```python
from build123d import *

# Parameters (mm, degrees)
SZKIC1_W                     = 24
SZKIC1_H                     = 52
DODANIE_WYCI_GNI_CIE1_DEPTH  = 25
SZKIC2_W                     = 26
SZKIC2_H                     = 54
SZKIC2_W_2                   = 21
SZKIC2_H_2                   = 49
DODANIE_WYCI_GNI_CIE2_DEPTH  = 12
SZKIC3_W                     = 38
SZKIC3_H                     = 54
SZKIC3_W_2                   = 21
SZKIC3_H_2                   = 49
DODANIE_WYCI_GNI_CIE3_DEPTH  = 2
SZKIC4_W                     = 38
SZKIC4_H                     = 54
DODANIE_WYCI_GNI_CIE4_DEPTH  = 3
ZAOKR_GLENIE1_R              = 3.5
SZKIC5_R                     = 1.5
DODANIE_WYCI_GNI_CIE9_DEPTH  = 3
WYTNIJ_WYCI_GNI_CIE2_REACH   = 63.425
SZKIC7_W                     = 20
SZKIC7_H                     = 11
SZKIC8_W                     = 34
SZKIC8_H                     = 96
SZKIC8_W_2                   = 30
SZKIC8_H_2                   = 92
DODANIE_WYCI_GNI_CIE5_DEPTH  = 18.5
SZKIC9_W                     = 34
SZKIC9_H                     = 96
DODANIE_WYCI_GNI_CIE6_DEPTH  = 3
SZKIC10_R                    = 1.9
WYTNIJ_WYCI_GNI_CIE3_DEPTH   = 70.873099259
ZAOKR_GLENIE2_R              = 4
SZKIC11_W                    = 34
SZKIC11_H                    = 96
SZKIC11_R                    = 4
DODANIE_WYCI_GNI_CIE7_DEPTH  = 3.5
SZKIC20_R                    = 4
DODANIE_WYCI_GNI_CIE10_DEPTH = 10
SZKIC21_R                    = 4
DODANIE_WYCI_GNI_CIE11_DEPTH = 5
SZKIC13_R                    = 1.5
WYTNIJ_WYCI_GNI_CIE4_DEPTH   = 6
WYTNIJ_WYCI_GNI_CIE5_DEPTH   = 72.028163428
SFAZOWANIE1_SIZE             = 0.5
SFAZOWANIE2_SIZE             = 2.1
ZAOKR_GLENIE3_R              = 6
ZAOKR_GLENIE4_R              = 4
SZKIC18_R                    = 3.5
WYTNIJ_WYCI_GNI_CIE8_DEPTH   = 10
SFAZOWANIE3_SIZE             = 1.5
SZKIC19_R                    = 2
WYTNIJ_WYCI_GNI_CIE9_DEPTH   = 73.938330286
WYTNIJ_WYCI_GNI_CIE10_REACH  = 92.161
SZKIC22_W                    = 15
SZKIC22_H                    = 9
ZAOKR_GLENIE5_R              = 3


with BuildPart() as part:
    # Szkic1 → Dodanie-wyciągnięcie1 (new body)
    with BuildSketch(Plane(origin=(0, 0, 0), x_dir=(1, 0, 0), z_dir=(0, 1, 0))):
        Rectangle(SZKIC1_W, SZKIC1_H)
        with BuildLine():
            Line((10, 14.5), (10, -14.5))
            ThreePointArc((10, -14.5), (0, -24.5), (-10, -14.5))
            Line((-10, -14.5), (-10, 14.5))
            ThreePointArc((-10, 14.5), (0, 24.5), (10, 14.5))
        make_face(mode=Mode.SUBTRACT)
    extrude(amount=DODANIE_WYCI_GNI_CIE1_DEPTH)

    # Szkic2 → Dodanie-wyciągnięcie2 (add)
    with BuildSketch(Plane(origin=(0, 25, 0), x_dir=(1, 0, 0), z_dir=(0, 1, 0))):
        Rectangle(SZKIC2_W, SZKIC2_H)
        Rectangle(SZKIC2_W_2, SZKIC2_H_2, mode=Mode.SUBTRACT)
    extrude(amount=DODANIE_WYCI_GNI_CIE2_DEPTH)

    # Szkic3 → Dodanie-wyciągnięcie3 (add)
    with BuildSketch(Plane(origin=(0, 37, 0), x_dir=(1, 0, 0), z_dir=(0, 1, 0))):
        Rectangle(SZKIC3_W, SZKIC3_H)
        Rectangle(SZKIC3_W_2, SZKIC3_H_2, mode=Mode.SUBTRACT)
    extrude(amount=-DODANIE_WYCI_GNI_CIE3_DEPTH)

    # Szkic4 → Dodanie-wyciągnięcie4 (add)
    with BuildSketch(Plane(origin=(0, 37, 0), x_dir=(1, 0, 0), z_dir=(0, 1, 0))):
        Rectangle(SZKIC4_W, SZKIC4_H)
        Polygon((-10, 24.5), (10, 24.5), (10.5, 24.5), (10.5, 18.35), (18, 18.35), (18, 10.35), (10.5, 10.35), (10.5, -10.35), (18, -10.35), (18, -18.35), (10.5, -18.35), (10.5, -24.5), (10, -24.5), (-10, -24.5), (-10.5, -24.5), (-10.5, -18.35), (-18, -18.35), (-18, -10.35), (-10.5, -10.35), (-10.5, 10.35), (-18, 10.35), (-18, 18.35), (-10.5, 18.35), (-10.5, 24.5), align=None, mode=Mode.SUBTRACT)
    extrude(amount=DODANIE_WYCI_GNI_CIE4_DEPTH)

    # Zaokrąglenie1
    zaokr_glenie1_edges = [part.edges().sort_by_distance(p)[0] for p in [
        (10.5, 38.5, -18.35),
        (18, 38.5, -18.35),
        (18, 38.5, -10.35),
        (10.5, 38.5, -10.35),
        (10.5, 38.5, 10.35),
        (18, 38.5, 10.35),
        (18, 38.5, 18.35),
        (10.5, 38.5, 18.35),
        (-10.5, 38.5, 18.35),
        (-18, 38.5, 18.35),
        (-18, 38.5, 10.35),
        (-10.5, 38.5, 10.35),
        (-10.5, 38.5, -10.35),
        (-18, 38.5, -10.35),
        (-18, 38.5, -18.35),
        (-10.5, 38.5, -18.35),
    ]]
    fillet(zaokr_glenie1_edges, radius=ZAOKR_GLENIE1_R)

    # Szkic5 → Dodanie-wyciągnięcie9 (add)
    with BuildSketch(Plane(origin=(0, 37, 0), x_dir=(1, 0, 0), z_dir=(0, 1, 0))):
        with Locations(Location((13.85, -14.35, 0), (0, 0, 270))):
            Circle(SZKIC5_R)
        with Locations(Location((13.85, 14.35, 0), (0, 0, 270))):
            Circle(SZKIC5_R)
        with Locations(Location((-13.85, -14.35, 0), (0, 0, 90))):
            Circle(SZKIC5_R)
        with Locations(Location((-13.85, 14.35, 0), (0, 0, 90))):
            Circle(SZKIC5_R)
    extrude(amount=DODANIE_WYCI_GNI_CIE9_DEPTH)

    # Szkic7 → Wytnij-wyciągnięcie2 (cut, up to next)
    with BuildSketch(Plane.ZY.offset(19), mode=Mode.PRIVATE) as wytnij_wyci_gni_cie2_sk1:
        with Locations((0, 32)):
            Rectangle(SZKIC7_W, SZKIC7_H)
    wytnij_wyci_gni_cie2_tool1 = extrude(wytnij_wyci_gni_cie2_sk1.sketch, amount=-WYTNIJ_WYCI_GNI_CIE2_REACH, mode=Mode.PRIVATE) & part.part
    add(wytnij_wyci_gni_cie2_tool1.solids().sort_by_distance((-19, 32, 0))[0], mode=Mode.SUBTRACT)

    # Szkic8 → Dodanie-wyciągnięcie5 (add)
    with BuildSketch(Plane(origin=(0, 0, 0), x_dir=(1, 0, 0), z_dir=(0, 1, 0))):
        with Locations((29, 0)):
            Rectangle(SZKIC8_W, SZKIC8_H)
        with Locations((29, 0)):
            Rectangle(SZKIC8_W_2, SZKIC8_H_2, mode=Mode.SUBTRACT)
    extrude(amount=DODANIE_WYCI_GNI_CIE5_DEPTH)

    # Szkic9 → Dodanie-wyciągnięcie6 (add)
    with BuildSketch(Plane(origin=(0, 18.5, 0), x_dir=(1, 0, 0), z_dir=(0, 1, 0))):
        with Locations((29, 0)):
            Rectangle(SZKIC9_W, SZKIC9_H)
    extrude(amount=DODANIE_WYCI_GNI_CIE6_DEPTH)

    # Szkic10 → Wytnij-wyciągnięcie3 (cut, through all)
    with BuildSketch(Plane(origin=(0, 21.5, 0), x_dir=(1, 0, 0), z_dir=(0, 1, 0))):
        with Locations(Location((24.5, 37.5, 0), (0, 0, 270))):
            Circle(SZKIC10_R)
        with Locations(Location((24.5, -37.5, 0), (0, 0, 270))):
            Circle(SZKIC10_R)
    extrude(amount=-WYTNIJ_WYCI_GNI_CIE3_DEPTH, mode=Mode.SUBTRACT)

    # Zaokrąglenie2
    zaokr_glenie2_edges = [part.edges().sort_by_distance(p)[0] for p in [
        (44, 9.25, -46),
        (14, 9.25, -46),
        (14, 9.25, 46),
        (44, 9.25, 46),
    ]]
    fillet(zaokr_glenie2_edges, radius=ZAOKR_GLENIE2_R)

    # Szkic11 → Dodanie-wyciągnięcie7 (add)
    with BuildSketch(Plane(origin=(0, 21.5, 0), x_dir=(1, 0, 0), z_dir=(0, 1, 0))):
        with Locations((29, 0)):
            Rectangle(SZKIC11_W, SZKIC11_H)
        with Locations(Location((24.5, 37.5, 0), (0, 0, 90))):
            Circle(SZKIC11_R, mode=Mode.SUBTRACT)
        with Locations(Location((24.5, -37.5, 0), (0, 0, 90))):
            Circle(SZKIC11_R, mode=Mode.SUBTRACT)
    extrude(amount=DODANIE_WYCI_GNI_CIE7_DEPTH)

    # Szkic20 → Dodanie-wyciągnięcie10 (add)
    with BuildSketch(Plane(origin=(0, 25, 0), x_dir=(1, 0, 0), z_dir=(0, 1, 0))):
        Polygon((12, 27), (13, 27), (13, -27), (12, -27), (12, -48), (46, -48), (46, 48), (12, 48), align=None)
        with Locations(Location((24.5, 37.5, 0), (0, 0, 90))):
            Circle(SZKIC20_R, mode=Mode.SUBTRACT)
        with Locations(Location((24.5, -37.5, 0), (0, 0, 90))):
            Circle(SZKIC20_R, mode=Mode.SUBTRACT)
    extrude(amount=DODANIE_WYCI_GNI_CIE10_DEPTH)

    # Szkic21 → Dodanie-wyciągnięcie11 (add)
    with BuildSketch(Plane(origin=(0, 35, 0), x_dir=(1, 0, 0), z_dir=(0, 1, 0))):
        Polygon((12, 27), (19, 27), (19, -27), (12, -27), (12, -48), (46, -48), (46, 48), (12, 48), align=None)
        with Locations(Location((24.5, 37.5, 0), (0, 0, 90))):
            Circle(SZKIC21_R, mode=Mode.SUBTRACT)
        with Locations(Location((24.5, -37.5, 0), (0, 0, 90))):
            Circle(SZKIC21_R, mode=Mode.SUBTRACT)
    extrude(amount=DODANIE_WYCI_GNI_CIE11_DEPTH)

    # Szkic13 → Wytnij-wyciągnięcie4 (cut)
    with BuildSketch(Plane(origin=(0, 40, 0), x_dir=(1, 0, 0), z_dir=(0, 1, 0))):
        with Locations(Location((41.5, 33, 0), (0, 0, 270))):
            Circle(SZKIC13_R)
        with Locations(Location((41.5, -33, 0), (0, 0, 270))):
            Circle(SZKIC13_R)
        with Locations(Location((16.5, -33, 0), (0, 0, 90))):
            Circle(SZKIC13_R)
        with Locations(Location((16.5, 33, 0), (0, 0, 90))):
            Circle(SZKIC13_R)
        with Locations(Location((29, 0, 0), (0, 0, 270))):
            Circle(SZKIC13_R)
    extrude(amount=-WYTNIJ_WYCI_GNI_CIE4_DEPTH, mode=Mode.SUBTRACT)

    # Szkic14 → Wytnij-wyciągnięcie5 (cut, through all)
    with BuildSketch(Plane(origin=(0, 25, 0), x_dir=(1, 0, 0), z_dir=(0, 1, 0))):
        Polygon((10, 0), (10, 18.642135624), (4.142135624, 24.5), (-4.142135624, 24.5), (-10, 18.642135624), (-10, 0), (-10, -18.642135624), (-4.142135624, -24.5), (4.142135624, -24.5), (10, -18.642135624), align=None)
    extrude(amount=-WYTNIJ_WYCI_GNI_CIE5_DEPTH, mode=Mode.SUBTRACT)

    # Sfazowanie1
    sfazowanie1_edges = [part.edges().sort_by_distance(p)[0] for p in [
        (10.5, 25, 0),
        (-10.5, 25, 0),
    ]]
    chamfer(sfazowanie1_edges, length=SFAZOWANIE1_SIZE - 0.0001)  # a hair under: the kernel refuses the full size

    # Sfazowanie2
    sfazowanie2_edges = [part.edges().sort_by_distance(p)[0] for p in [
        (24.5, 21.5, -33.5),
        (24.5, 21.5, 41.5),
    ]]
    chamfer(sfazowanie2_edges, length=SFAZOWANIE2_SIZE - 0.0001)  # a hair under: the kernel refuses the full size

    # Zaokrąglenie3
    zaokr_glenie3_edges = [part.edges().sort_by_distance(p)[0] for p in [
        (12, 12.5, 26),
        (12, 12.5, -26),
        (-19, 37.5, 27),
        (-19, 37.5, -27),
        (-12, 12.5, -26),
        (-12, 12.5, 26),
        (12, 20, -48),
        (46, 20, -48),
        (46, 20, 48),
        (12, 20, 48),
        (-13, 30, -27),
        (-13, 30, 27),
    ]]
    fillet(zaokr_glenie3_edges, radius=ZAOKR_GLENIE3_R)

    # Zaokrąglenie4
    zaokr_glenie4_edges = [part.edges().sort_by_distance(p)[0] for p in [
        (-15.737192685, 37.5, 10),
        (-15.737192685, 37.5, -10),
    ]]
    fillet(zaokr_glenie4_edges, radius=ZAOKR_GLENIE4_R)

    # Szkic18 → Wytnij-wyciągnięcie8 (cut)
    with BuildSketch(Plane(origin=(0, 40, 0), x_dir=(1, 0, 0), z_dir=(0, 1, 0))):
        with Locations((47, 40)):
            Circle(SZKIC18_R)
        with Locations((47, -40)):
            Circle(SZKIC18_R)
    extrude(amount=-WYTNIJ_WYCI_GNI_CIE8_DEPTH, mode=Mode.SUBTRACT)

    # Sfazowanie3
    sfazowanie3_edges = [part.edges().sort_by_distance(p)[0] for p in [
        (43.500820064, 30, -39.924238715),
        (43.500820064, 30, 39.924238715),
    ]]
    chamfer(sfazowanie3_edges, length=SFAZOWANIE3_SIZE)

    # Szkic19 → Wytnij-wyciągnięcie9 (cut, through all)
    with BuildSketch(Plane(origin=(0, 30, 0), x_dir=(1, 0, 0), z_dir=(0, 1, 0))):
        with Locations((47, -40)):
            Circle(SZKIC19_R)
        with Locations((47, 40)):
            Circle(SZKIC19_R)
    extrude(amount=-WYTNIJ_WYCI_GNI_CIE9_DEPTH, mode=Mode.SUBTRACT)

    # Szkic22 → Wytnij-wyciągnięcie10 (cut, up to next)
    with BuildSketch(Plane(origin=(46, 0, 0), x_dir=(0, 0, -1), z_dir=(1, 0, 0)), mode=Mode.PRIVATE) as wytnij_wyci_gni_cie10_sk1:
        with Locations((15.5, 6.7)):
            Rectangle(SZKIC22_W, SZKIC22_H)
    wytnij_wyci_gni_cie10_tool1 = extrude(wytnij_wyci_gni_cie10_sk1.sketch, amount=-WYTNIJ_WYCI_GNI_CIE10_REACH, mode=Mode.PRIVATE) & part.part
    add(wytnij_wyci_gni_cie10_tool1.solids().sort_by_distance((46, 6.7, -15.5))[0], mode=Mode.SUBTRACT)

    # Zaokrąglenie5
    zaokr_glenie5_edges = [part.edges().sort_by_distance(p)[0] for p in [
        (45, 2.2, -8),
        (45, 11.2, -8),
        (45, 11.2, -23),
        (45, 2.2, -23),
    ]]
    fillet(zaokr_glenie5_edges, radius=ZAOKR_GLENIE5_R)


solid = part.part
```
Could you check a few things on this model? Use its own coordinates, in mm. A direction names the side the tool comes from. Round coordinates to 2 decimals unless told otherwise and drop trailing zeros. Loops run counter-clockwise (first coordinate to the right, second up) from the corner with the lowest first, then second, coordinate; pieces in that order, holes last.
Q1. On a 3-axis mill with a long thin cutter (end or side, diameter ignored), from which of +Z, -Z, +X, -X, +Y, -Y can I reach the whole of each face in a straight line? I mean faces 1 (the cylindrical face through (44.99, 3.1, -8.86)), 2 (the cylindrical face through (11.5, 38.5, -19.4)), 3 (the flat face through (-13, 25.5, 0.3)), 4 (the flat face through (-7.11, 12.68, 21.53)), 5 (the cylindrical face through (-11.196, 30.07, 25.289)). Say none if no direction works.
Q2. I want a section at D-D (z = 23.5). Write out the boundary of the cut face in (x, y), and give its area (3 significant figures).
Q3. I want a section at B-B (z = -0.5). Give the number of separate pieces and of enclosed holes in the cut face, and give its area (3 significant figures).
Q4. Please list where these lines run through material, in increasing order: L1, parallel to Z at x = 24.5, y = 32.75; L2, parallel to X at y = 37.75, z = -33; L3, parallel to Z at x = 18.5, y = 12.5.
Q5. Thinking about a two-plate mould opening in X: for faces 6 (the cylindrical face through (-17.196, 37.465, -25.289)), 7 (the flat face through (-12, 30, 10)), 8 (the cylindrical face through (16.43, 37.04, -31.5)), which applies, pulls with the +X half, pulls with the -X half, needs draft (parallel to the pull), parting line crosses it, or undercut?
Q6. For P1, Ø1.5, axis at x = 2.5, y = 31.5, coming from the +Z side; P2, Ø11, axis at y = 29.5, z = -2.5, coming from the -X side; P3, Ø10, axis at x = 0, y = 19.5, coming from the -Z side, each with a flat end and sliding along its axis, tell me the tip position at first contact or that it passes through.
Q7. I want a section at A-A (x = -1). Write out the boundary of the cut face in (y, z), and give its area (3 significant figures).
Answer below:
1. face 1: +X
1. face 2: +Y
1. face 3: +Z, -Z, -X, -Y
1. face 4: +Y, -Y
1. face 5: +Z, -X, -Y
2. outline: (-18.45, 35) - (-12.45, 35) - (-12.45, 25) - (-10.87, 25) - (-10.87, 0) - (-5.14, 0) - (-5.14, 25) - (-10, 25) - (-10.5, 25.5) - (-10.5, 40) - (-18.45, 40) - close; (5.14, 0) - (14, 0) - (14, 18.5) - (44, 18.5) - (44, 0) - (46, 0) - (46, 40) - (10.5, 40) - (10.5, 25.5) - (10, 25) - (5.14, 25) - close
2. area: 1,200 mm2
3. separate pieces: 3
3. enclosed holes: 0
3. area: 936 mm2
4. L1: z = -48 to -41.5, -33.5 to 33.5, 41.5 to 48
4. L2: x = 12 to 15, 18 to 40, 43 to 46
4. L3: z = -48 to -46, 46 to 48
5. face 6: pulls with the -X half
5. face 7: needs draft
5. face 8: undercut
6. P1: stops at z = 27
6. P2: stops at x = -13
6. P3: stops at z = -26
7. outline: (0, -26) - (25, -26) - (25, -27) - (40, -27) - (40, -24.5) - (0, -24.5) - close; (0, 24.5) - (40, 24.5) - (40, 27) - (25, 27) - (25, 26) - (0, 26) - close
7. area: 150 mm2
